from build123d import *

# Parameters (mm, degrees)
ESQUISSE1_W             = 40
ESQUISSE1_H             = 43
BOSS_EXTRU_1_DEPTH      = 12
ESQUISSE2_R             = 2.5
ENL_V_MAT_EXTRU_1_DEPTH = 60.941638283
CONG_1_R                = 4


with BuildPart() as part:
    # Esquisse1 → Boss.-Extru.1 (new body)
    with BuildSketch(Plane.XY):
        with Locations((20, 21.5)):
            Rectangle(ESQUISSE1_W, ESQUISSE1_H)
    extrude(amount=BOSS_EXTRU_1_DEPTH)

    # Esquisse2 → Enlèv. mat.-Extru.1 (cut, through all)
    with BuildSketch(Plane.XY.offset(12)):
        with Locations((10, 30)):
            Circle(ESQUISSE2_R)
        with Locations(Location((10, 10, 0), (0, 0, 180))):
            Circle(ESQUISSE2_R)
        with Locations((30, 10)):
            Circle(ESQUISSE2_R)
        with Locations(Location((30, 30, 0), (0, 0, 180))):
            Circle(ESQUISSE2_R)
    extrude(amount=-ENL_V_MAT_EXTRU_1_DEPTH, mode=Mode.SUBTRACT)

    # Congé1
    cong_1_edges = [part.edges().sort_by_distance(p)[0] for p in [
        (0, 43, 6),
        (40, 43, 6),
        (40, 0, 6),
        (0, 0, 6),
    ]]
    fillet(cong_1_edges, radius=CONG_1_R)


solid = part.part
Verification items for the finished model (mm, model axes). Coordinates: 2 decimals unless noted, no trailing zeros. Order: outer loops, then holes, each group sorted by start corner. A loop starts at its lowest first (then second) coordinate and runs counter-clockwise, first axis right, second up. Notation, with made-up numbers: M 84,-8 L 125,-8 A15 cw 125,18 Z; hole C 23,-25 d7. An arc over 180 degrees is marked long. Write each question's results on one line, items separated by ' | '.
1) Section check B-B on x = 10. Record the cut outline in (y, z), plus the area to 3 significant figures.
Solved:
outline: M 0,0 L 7.5,0 L 7.5,12 L 0,12 Z; M 12.5,0 L 27.5,0 L 27.5,12 L 12.5,12 Z; M 32.5,0 L 43,0 L 43,12 L 32.5,12 Z | area: 396 mm²
2) Scan lines: line 1 along Y through (x, z) = (10, 5); line 2 along Y through (x, z) = (8, 3.25); line 3 along X through (y, z) = (8, 10.25). Record each from-to range of solid material in increasing order. Write a range as [from, to].
Solved:
line 1: y = [0, 7.5], [12.5, 27.5], [32.5, 43] | line 2: y = [0, 8.5], [11.5, 28.5], [31.5, 43] | line 3: x = [0, 8.5], [11.5, 28.5], [31.5, 40]
3) Release check for a two-part mould opening along Y. For faces 1 (the face through (11.34, 32.11, 6.08)), 2 (the face through (40, 21, 6)), 3 (the face through (1.141, 41.797, 6.084)) record: pulls with the +Y half, pulls with the -Y half, needs draft (parallel to the pull), parting line crosses it, or undercut.
Solved:
face 1: undercut | face 2: needs draft | face 3: pulls with the +Y half
4) Section check A-A on y = 30. Record the cut outline in (x, z), plus the area to 3 significant figures.
Solved:
outline: M 0,0 L 7.5,0 L 7.5,12 L 0,12 Z; M 12.5,0 L 27.5,0 L 27.5,12 L 12.5,12 Z; M 32.5,0 L 40,0 L 40,12 L 32.5,12 Z | area: 360 mm²
5) Section check C-C on z = 2.5. Record the cut outline in (x, y), plus the area to 3 significant figures.
Solved:
outline: M 0,4 A4 ccw 4,0 L 36,0 A4 ccw 40,4 L 40,39 A4 ccw 36,43 L 4,43 A4 ccw 0,39 Z; hole C 10,10 d5; hole C 10,30 d5; hole C 30,10 d5; hole C 30,30 d5 | area: 1,630 mm²
